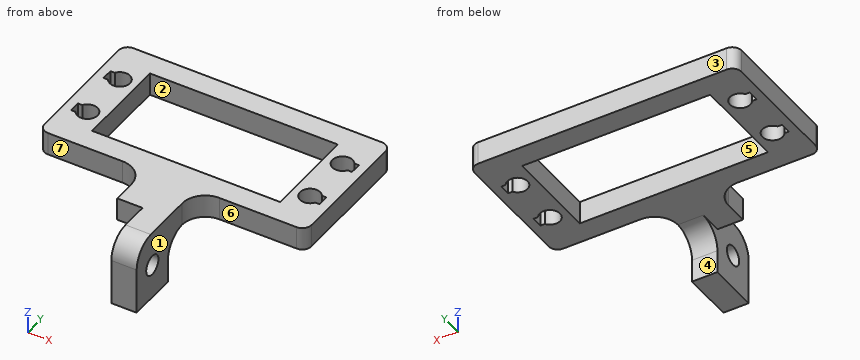
Autodesk Inventor part; units mm, degrees
ref_plane "Work Plane1" through (20.15, 10, -1.65) normal (-1, 0, 0) x (0, 1, 0)
ref_plane "YZ Plane" through (0, 0, 0) normal (1, 0, 0) x (0, 1, 0)
ref_plane "XZ Plane" through (0, 0, 0) normal (0, 1, 0) x (-1, 0, 0)
sketch "Sketch1" plane through (0, 0, 0) normal (0, 0, 1) x (1, 0, 0)
  line L0 (0, 0) -> (-6.8, 0)
  line L1 (-6.8, 0) -> (-6.8, 20)
  line L2 (-6.8, 20) -> (0, 20)
  line L3 (0, 20) -> (0, 0)
  line L4 (-5.8439, 5.5) -> (-6.8, 5.5)
  line L5 (-6.8, 14.5) -> (-6.8, 5.5)
  line L6 (-6.8, 14.5) -> (-5.8439, 14.5)
  arc A0 (-5.8439, 14.5) -> (-5.8439, 16.9) centre (-4, 15.7) ccw
  line L7 (-5.8439, 16.9) -> (-6.8, 16.9)
  line L8 (-6.8, 20) -> (-6.8, 16.9)
  line L9 (0, 20) -> (-6.8, 20)
  line L10 (0, 0) -> (0, 20)
  line L11 (0, 0) -> (-6.8, 0)
  line L12 (-6.8, 3.1) -> (-6.8, 0)
  line L13 (-6.8, 3.1) -> (-5.8439, 3.1)
  arc A1 (-5.8439, 3.1) -> (-5.8439, 5.5) centre (-4, 4.3) ccw
  dimension "d0" = 6.8
  dimension "d1" = 20
extrude "Extrusion1" add sketch "Sketch1" along normal blind 5 contours L0 L1 L13 A1 L4 L6 A0 L7 L2 L3
ref_plane "Work Plane1" through (20.15, 10, -1.65) normal (-1, 0, 0) x (0, 1, 0)
mirror "Mirror1" about plane through (20.15, 10, -1.65) normal (-1, 0, 0) of "Extrusion1"
sketch "Sketch2" plane through (-6.8, 0, 0) normal (0, -1, 0) x (1, 0, 0)
  line L0 (0, 0) -> (53.9, 0)
  line L1 (53.9, 0) -> (53.9, 5)
  line L2 (53.9, 5) -> (0, 5)
  line L3 (0, 5) -> (0, 0)
  dimension "d4" = 53.9
extrude "Extrusion2" add sketch "Sketch2" along normal blind 5
sketch "Sketch3" plane through (-6.8, 3.1, 0) normal (-1, 0, 0) x (0, 0, 1)
  line L0 (0, -8.1) -> (5, -8.1)
  line L1 (5, -8.1) -> (5, 16.9)
  line L2 (5, 16.9) -> (0, 16.9)
  line L3 (0, 16.9) -> (0, -8.1)
  point P0 (0, -3.1)
  dimension "d7" = 25
extrude "Extrusion3" add sketch "Sketch3" along normal blind 2
mirror "Mirror2" about plane through (20.15, 10, -1.65) normal (-1, 0, 0) of "Extrusion3"
fillet "Fillet1" radius 2 1 edges at (-8.8, -5, 2.5)
fillet "Fillet2" radius 2 1 edges at (49.1, -5, 2.5)
sketch "Sketch4" plane through (0, 20, 5) normal (1, 0, 0) x (0, 0, -1)
  line L0 (5, -20) -> (5, 0)
  line L1 (5, 0) -> (0, 0)
  line L2 (0, -20) -> (0, 0)
  line L3 (5, -20) -> (0, -20)
extrude "Extrusion4" cut sketch "Sketch4" against normal blind 0.25
mirror "Mirror3" about plane through (20.15, 10, -1.65) normal (-1, 0, 0) of "Extrusion4"
sketch "Sketch5" plane through (-8.8, 20, 5) normal (0, 1, 0) x (1, 0, 0)
  line L0 (0, 0) -> (57.9, 0)
  line L1 (57.9, 0) -> (57.9, 5)
  line L2 (57.9, 5) -> (0, 5)
  line L3 (0, 5) -> (0, 0)
  point P0 (8.8, 5)
  dimension "d14" = 57.9
extrude "Extrusion5" add sketch "Sketch5" along normal blind 5
sketch "Sketch6" plane through (-8.8, 20, 5) normal (0, -1, 0) x (1, 0, 0)
  line L0 (8.55, 0) -> (8.55, -5)
  line L1 (49.35, -5) -> (8.55, -5)
  line L2 (49.35, -5) -> (49.35, 0)
  line L3 (8.55, 0) -> (49.35, 0)
  point P0 (8.8, -5)
extrude "Extrusion6" cut sketch "Sketch6" against normal blind 0.15
sketch "Sketch7" plane through (-6.8, 0, 0) normal (0, 1, 0) x (1, 0, 0)
  line L0 (47.35, -5) -> (6.55, -5)
  line L1 (47.35, 0) -> (47.35, -5)
  line L2 (6.55, 0) -> (47.35, 0)
  line L3 (6.55, 0) -> (6.55, -5)
  point P0 (6.8, 0)
extrude "Extrusion7" cut sketch "Sketch7" against normal blind 0.15
sketch "Sketch9" plane through (-6.8, -5, 0) normal (0, -1, 0) x (1, 0, 0)
  line L0 (0, 5) -> (53.9, 5)
  line L1 (53.9, 0) -> (0, 0)
  line L2 (26.65, -10.0707) -> (26.65, 15.0707) construction
  line L3 (55.9, 0) -> (55.9, 5) construction
  line L4 (21.15, 5) -> (32.15, 5)
  line L5 (32.15, 5) -> (32.15, 0)
  line L6 (32.15, 0) -> (21.15, 0)
  line L7 (21.15, 0) -> (21.15, 5)
  point P0 (6.8, 0)
  dimension "d23" = 29.25
  dimension "d24" = 11
  dimension "d25" = 5.5
extrude "Extrusion9" add sketch "Sketch9" along normal blind 21
fillet "Fillet3" radius 5 2 edges at (14.35, -5, 2.5) (25.35, -5, 2.5)
sketch "Sketch10" plane through (0, 0, 0) normal (0, 0, -1) x (-1, 0, 0)
  line L0 (-47.1, -5) -> (-30.35, -5)
  line L1 (-14.35, -10) -> (-14.35, -26)
  line L2 (-25.35, -15) -> (-19.85, -15)
  line L3 (-19.85, -15) -> (-19.85, -26)
  line L4 (-19.85, -26) -> (-25.35, -26)
  line L5 (-25.35, -10) -> (-25.35, -26)
  line L6 (-9.35, -5) -> (6.8, -5)
  line L7 (-25.35, -15) -> (-25.35, -26)
  point P0 (0, 0)
  dimension "d30" = 11
  dimension "d31" = 10
  dimension "d32" = 5.5
extrude "Extrusion10" add sketch "Sketch10" along normal blind 10
fillet "Fillet7" radius 5 1 edges at (22.6, -15, 0)
sketch "Sketch11" plane through (0, 0, 0) normal (0, 0, -1) x (-1, 0, 0)
  line L0 (-19.85, -10) -> (-19.85, -26)
  line L1 (-14.35, -26) -> (-19.85, -26)
  line L2 (-19.85, -26) -> (-19.85, -15)
  line L3 (-19.85, -15) -> (-14.35, -15)
  line L4 (-14.35, -15) -> (-14.35, -26)
  point P0 (0, 0)
  dimension "d39" = 11
extrude "Extrusion11" cut sketch "Sketch11" against normal blind 10
sketch "Sketch12" plane through (25.35, -26, 5) normal (1, 0, 0) x (0, 0, -1)
  line L0 (15, 11) -> (15, 0)
  circle A0 centre (7.5, 5.5) radius 2.15
  point P0 (5, 26)
  dimension "d42" = 4.3
  dimension "d43" = 7.5
extrude "Extrusion12" cut sketch "Sketch12" against normal blind 10
fillet "Fillet8" radius 5 1 edges at (22.6, -26, 5)
sketch "Sketch14" plane through (20.15, 10, -1.65) normal (1, 0, 0) x (0, 1, 0)
  point P0 (-10, -1.65)
fillet "Fillet9" radius 2 2 edges at (49.1, 25, 2.5) (-8.8, 25, 2.5)
ref_plane "Work Plane2" through (20.15, 10, -1.65) normal (-1, 0, 0) x (0, 1, 0)
properties part number "TopBar"
The model under review builds one solid part; all positions refer to its coordinate system, in mm. Face numbers are marked on the shaded views. A direction names the side the tool comes from. Coordinates: 2 decimals unless noted, no trailing zeros. Write each loop counter-clockwise with the first axis right and the second up, starting at its lowest first coordinate (ties: lowest second). Pieces come first, ordered by that corner, then holes.
1) We need section B-B on x = 8. State the section outline as (y, z) points, then the cut area to 3 significant figures.
2) Clearance check with flat-ended pins moving along their axes: pin 1 Ø6 at (x, z) = (35, 2.5) entering from -Y; pin 2 Ø5.5 at (x, z) = (16, 3) entering from -Y; pin 3 Ø2.5 at (x, z) = (21.5, -7.5) entering from +Y. State where each tip first meets the part, or that it passes through.
3) To check wall thickness, follow probe 1 along Y at (x, z) = (-4, 2.5); probe 2 along X at (y, z) = (4.3, 3.05); probe 3 along Y at (x, z) = (9, 3.5). State the ranges of each line that lie inside material, in increasing order.
4) We need section A-A on y = 7.5. State the section outline as (x, z) points.
5) The part is to be moulded in two halves that separate along X. For the marked faces 1, 2 and 3, say which applies: pulls with the +X half, pulls with the -X half, needs draft (parallel to the pull), parting line crosses it, or undercut.
6) Machinability: for the marked faces 4, 5, 6 and 7, which of the approach directions +Z, -Z, +X, -X, +Y, -Y give a long, thin tool a straight path to every point of the face, cutting with its end or side? Answer none if there is none.
7) We need section C-C on y = 16. State the section outline as (x, z) points, then the cut area to 3 significant figures.
Answer list:
1. outline: (-5, 0) - (-0.15, 0) - (-0.15, 5) - (-5, 5) - close; (20.15, 0) - (25, 0) - (25, 5) - (20.15, 5) - close
1. area: 48.5 mm2
2. pin 1: stops at y = -5
2. pin 2: stops at y = -15
2. pin 3: stops at y = -15
3. probe 1: y = -5 to 2.1, 6.5 to 13.5, 17.9 to 25
3. probe 2: x = -8.8 to -6.8, -1.8 to -0.25, 40.55 to 42.1, 47.1 to 49.1
3. probe 3: y = -5 to -0.15, 20.15 to 25
4. outline: (-8.8, 0) - (-0.25, 0) - (-0.25, 5) - (-8.8, 5) - close; (40.55, 0) - (49.1, 0) - (49.1, 5) - (40.55, 5) - close
5. face 1: pulls with the +X half
5. face 2: undercut
5. face 3: needs draft
6. face 4: -Z, +X, -X, +Y
6. face 5: +Z, -Z
6. face 6: +Z, -Z, +X, -Y
6. face 7: +Z, -Z, -X, -Y
7. outline: (-8.8, 0) - (-6.8, 0) - (-6.8, 5) - (-8.8, 5) - close; (-1.82, 0) - (-0.25, 0) - (-0.25, 5) - (-1.82, 5) - close; (40.55, 0) - (42.12, 0) - (42.12, 5) - (40.55, 5) - close; (47.1, 0) - (49.1, 0) - (49.1, 5) - (47.1, 5) - close
7. area: 35.7 mm2
